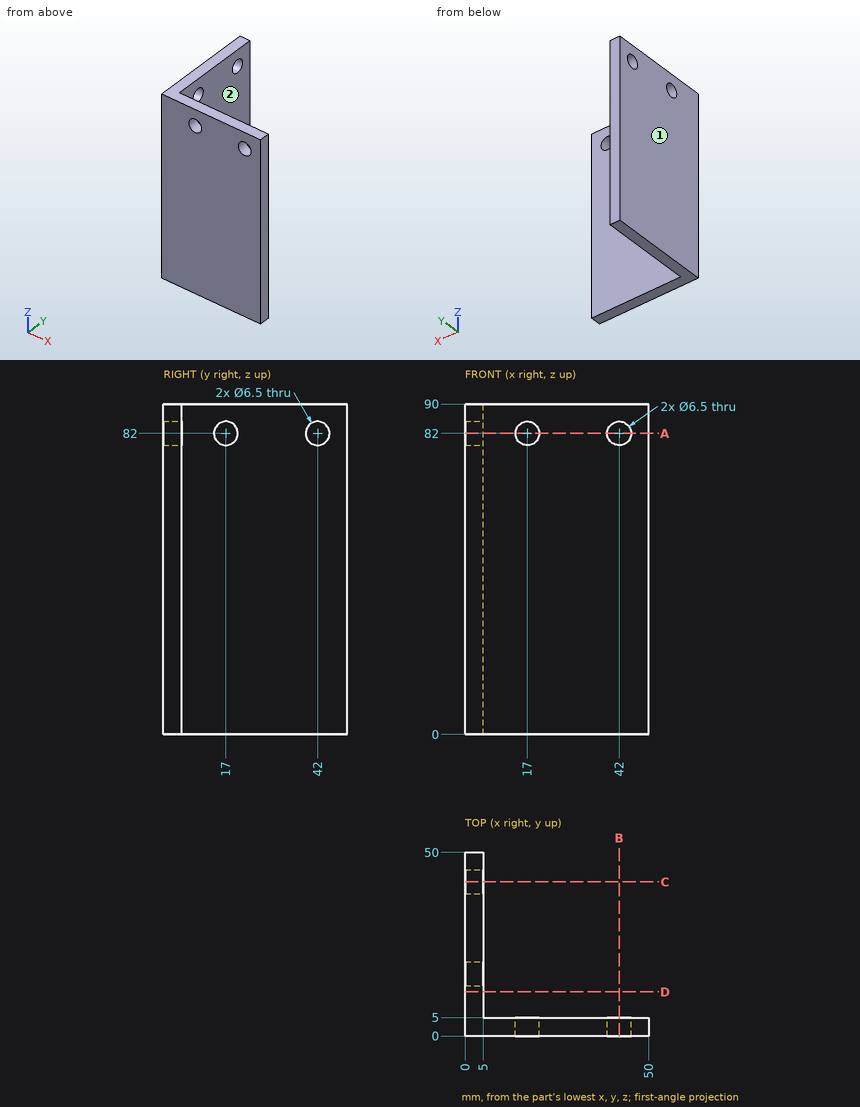
Geometry: see drawing. Coordinates: mm, zero at the bounding-box minimum. A direction names the side the tool comes from. Coordinates: 2 decimals unless noted, no trailing zeros. Loops run counter-clockwise (first coordinate to the right, second up) from the corner with the lowest first, then second, coordinate; pieces in that order, holes last. Notation, with made-up numbers: (38.5, 36.5) - (42.5, 36.5) arc R19 ccw to (42.5, 51.5) - close; hole circle Ø6 at (67.25, 49). An arc over 180 degrees is marked (long way). Answer as CSV lines item,"result".
1. Section B-B (x = 42). Return loops of the section in (y, z).
Established:
outline,"(0, 0) - (5, 0) - (5, 78.75) - (0, 78.75) - close; (0, 85.25) - (5, 85.25) - (5, 90) - (0, 90) - close"
2. Reachability of the marked faces 1 and 2 from +Z, -Z, +X, -X, +Y, -Y: full face, straight path, thin tool, end or side. Return the list, or none.
Established:
face 1,"+Z, -Z, -X, +Y, -Y"
face 2,"+Z, -Z, +X, +Y"
3. Contact query for flat-ended pins moving along their axis: pin 1 (12 mm diameter, centred on y = 38, z = 13, fed in from +X); pin 2 (8 mm diameter, centred on x = 36.5, y = 6.5, fed in from -Z); pin 3 (12 mm diameter, centred on x = 30, z = 76.5, fed in from +Y). Output: stop coordinate, or through.
Established:
pin 1,"stops at x = 5"
pin 2,"stops at z = 0"
pin 3,"stops at y = 5"
4. Ray query, line 1 (Y direction, x = 1, z = 82); line 2 (Z direction, x = 17, y = 2.4). Return the intervals inside material, ascending.
Established:
line 1,"y = 0 to 13.75, 20.25 to 38.75, 45.25 to 50"
line 2,"z = 0 to 78.75, 85.25 to 90"
5. Section D-D (y = 12). Return loops of the section in (x, z).
Established:
outline,"(0, 0) - (5, 0) - (5, 90) - (0, 90) - close"
6. Section A-A (z = 82). Return loops of the section in (x, y).
Established:
outline,"(0, 0) - (13.75, 0) - (13.75, 5) - (5, 5) - (5, 13.75) - (0, 13.75) - close; (0, 20.25) - (5, 20.25) - (5, 38.75) - (0, 38.75) - close; (0, 45.25) - (5, 45.25) - (5, 50) - (0, 50) - close; (20.25, 0) - (38.75, 0) - (38.75, 5) - (20.25, 5) - close; (45.25, 0) - (50, 0) - (50, 5) - (45.25, 5) - close"
